CAD build for the part. Positions are in the model's coordinates, mm. Round coordinates to 2 decimals unless told otherwise and drop trailing zeros. Loops run counter-clockwise (first coordinate to the right, second up) from the corner with the lowest first, then second, coordinate; pieces in that order, holes last.
Autodesk Inventor part; units mm, degrees
ref_plane "YZ Plane" through (0, 0, 0) normal (1, 0, 0) x (0, 1, 0)
ref_plane "XY Plane" through (0, 0, 0) normal (0, 0, 1) x (1, 0, 0)
ref_plane "Work Plane1" through (0, 0, 0) normal (0, 0, 1) x (1, 0, 0)
sketch "Sketch1" plane through (0, 0, 0) normal (0, 0, 1) x (1, 0, 0)
  line L0 (-58.0302, -14) -> (-60.5225, -14) construction
  line L1 (-54.7493, -17.6642) -> (-59.4824, 0)
  line L2 (-65.1814, 17.4053) -> (-55.7152, -17.923)
  line L3 (-59.4824, 0) -> (-60.5176, 0) construction
  line L4 (-144, 0) -> (-60.5176, 0) construction
  line L5 (-47.8265, 0) -> (-82.556, 0) construction
  line L6 (-64.2155, 17.6642) -> (-65.1814, 17.4053)
  line L7 (-55.7152, -17.923) -> (-54.7493, -17.6642)
  line L8 (-59.4824, 0) -> (-64.2155, 17.6642)
  line L9 (-60.5176, 0) -> (24, 0) construction
  line L10 (-144, 0) -> (24, 0)
  line L11 (-60, 54.8295) -> (-60, -83.9771)
  point P0 (0, 0)
  point P1 (-60, 0)
  dimension "d2" = 1
  dimension "d28" = 17.6642
  dimension "d29" = 15
extrude "Extrusion1" add sketch "Sketch1" along normal blind 30 and the other way blind 30
ref_plane "Work Plane2" through (-60, 0, -16) normal (1, 0, 0) x (0, 0, -1)
sketch "Sketch2" plane through (-60, 0, -16) normal (1, 0, 0) x (0, 0, -1)
  circle A0 centre (-16, 0) radius 17.5
  dimension "d26" = 35
extrude "Extrusion2" cut sketch "Sketch2" along normal mid plane 30 keep common part
sketch "Sketch5" plane through (-60, 0, -16) normal (1, 0, 0) x (0, 0, -1)
  circle A0 centre (-16, 0) radius 14
  dimension "d30" = 28
extrude "Extrusion4" cut sketch "Sketch5" along normal mid plane 10 keep common part
sketch "Sketch7" plane through (-59.4824, 0, 0) normal (0.9659, 0.2588, 0) x (0, 0, -1)
  line L0 (-33.8, 0.134) -> (-42.2, 0.134) construction
  line L1 (-86, 0.134) -> (89, 0.134) construction
  line L2 (-86, 0.134) -> (89, 0.134) construction
  circle A0 centre (7.5, 0.134) radius 1.5 construction
  circle A1 centre (-7.5, 0.134) radius 1.5 construction
  line L3 (0, -21.4266) -> (0, 20.7932) construction
  point P0 (0, -15.3952)
  dimension "d34" = 3
  dimension "d35" = 7.5
  dimension "d36" = 7.5
hole "Hole2" at (-59.517, 0.1294, -7.5) at (-59.517, 0.1294, 7.5) direction (-0.9659, -0.2588, 0) diameter 3 end through all
properties part number "butterfly" material "Brass, Soft Yellow"
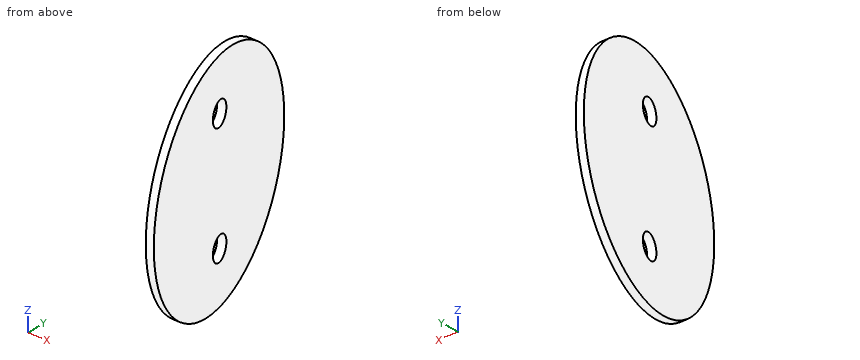
Item 1: Cut at A-A (z = 0). List the corners of the cut face in (x, y).
Verdict:
outline: (-64.27, 14) - (-56.77, -14) - (-55.73, -14) - (-63.23, 14) - close
Item 2: Wall check: L1, parallel to X at y = -7.25, z = -2.75; L2, parallel to X at y = 2.5, z = 6.5; L3, parallel to Z at x = -61, y = 5. Give the ranges that are in metal, low to high.
Verdict:
L1: x = -58.58 to -57.54
L2: x = -61.19 to -60.15
L3: z = -13.08 to 13.08
Item 3: Flat gauge pins, fed straight in: P1, Ø3, axis at x = -58.5, z = 7.5, coming from the -Y side; P2, Ø6, axis at y = 4, z = -2.5, coming from the -X side; P3, Ø6, axis at y = 10, z = -6.5, coming from the -X side. Where does each tip first touch, or does it go through?
Verdict:
P1: stops at y = -12.29
P2: stops at x = -62.39
P3: stops at x = -63.96
Item 4: Cut at B-B (x = -58.5). List the corners of the cut face in (y, z), plus the area to 3 significant figures.
Verdict:
outline: (-7.53, -11.8) arc R14 ccw to (-3.67, -13.51) - (-3.67, 13.51) arc R14 ccw to (-7.53, 11.8) - close
area: 98.7 mm2
